```python
from build123d import *

# Parameters (mm, degrees)
BOSS_EXTRUDE1_DEPTH     = 8
BOSS_EXTRUDE2_DEPTH     = 2
SKETCH3_R               = 2.05
CUT_EXTRUDE3_DEPTH      = 10
CUT_EXTRUDE3_DEPTH_BACK = 10
FILLET2_R               = 4
SKETCH6_R               = 7.5
BOSS_EXTRUDE3_DEPTH     = 6
SKETCH2_R               = 5.5
CUT_EXTRUDE4_DEPTH      = 28.361360249
CUT_EXTRUDE4_DEPTH_BACK = 3
SKETCH8_R               = 0.8
CUT_EXTRUDE5_DEPTH      = 30.928860828
FILLET3_R               = 3


with BuildPart() as part:
    # Sketch1 → Boss-Extrude1 (new body)
    with BuildSketch(Plane(origin=(0, 0, 0), x_dir=(1, 0, 0), z_dir=(0, 1, 0))):
        Polygon((0, 0), (0, 2), (26.334414729, 2), (34.518104392, -15.549979118), (32.760161227, -16.503727422), (25.996962058, -2), (21.605779457, -2), (21.605779457, 0), align=None)
    extrude(amount=BOSS_EXTRUDE1_DEPTH)

    # Sketch5 → Boss-Extrude2 (add)
    with BuildSketch(Plane(origin=(22.396969556, 0, -10.443878423), x_dir=(-0.422618262, 0, -0.906307787), z_dir=(0.906307787, 0, -0.422618262))):
        with BuildLine():
            Line((-40.780850255, 18.736062391), (-36.467218683, 26.428860828))
            ThreePointArc((-36.467218683, 26.428860828), (-23.692308478, 4.771999965), (-36.205658542, -17.037035395))
            Line((-36.205658542, -17.037035395), (-40.049339329, -9.057253488))
            ThreePointArc((-40.049339329, -9.057253488), (-32.517126315, 5.047276383), (-40.780850255, 18.736062391))
        make_face()
    extrude(amount=-BOSS_EXTRUDE2_DEPTH)

    # Sketch3 → Cut-Extrude3 (cut, two sides)
    with BuildSketch(Plane(origin=(20.587699136, 0, -9.600201771), x_dir=(0.422618262, 0, 0.906307787), z_dir=(-0.906307787, 0, 0.422618262))) as cut_extrude3_sk:
        with Locations((28.701516689, 4)):
            Circle(SKETCH3_R)
        with Locations((34.117040182, 18.317355913)):
            Circle(SKETCH3_R)
        with Locations((48.070293023, 24.611901983)):
            Circle(SKETCH3_R)
        with Locations((62.387648936, 19.19637849)):
            Circle(SKETCH3_R)
        with Locations((68.682195005, 5.243125649)):
            Circle(SKETCH3_R)
        with Locations((63.266671512, -9.074230264)):
            Circle(SKETCH3_R)
        with Locations((49.313418672, -15.368776333)):
            Circle(SKETCH3_R)
        with Locations((34.996062759, -9.953252841)):
            Circle(SKETCH3_R)
    extrude(amount=CUT_EXTRUDE3_DEPTH, mode=Mode.SUBTRACT)
    extrude(cut_extrude3_sk.sketch, amount=-CUT_EXTRUDE3_DEPTH_BACK, mode=Mode.SUBTRACT)

    # Fillet2
    fillet2_edges = [part.edges().sort_by_distance(p)[0] for p in [
        (31.687047343, 0, 11.840592477),
        (31.60186373, 8, 11.657915631),
    ]]
    fillet(fillet2_edges, radius=FILLET2_R)

    # Sketch6 → Boss-Extrude3 (add)
    with BuildSketch(Plane(origin=(0, 0, -2), x_dir=(-1, 0, 0), z_dir=(0, 0, -1))):
        with Locations((0, 4)):
            Circle(SKETCH6_R)
    extrude(amount=-BOSS_EXTRUDE3_DEPTH)

    # Sketch2 → Cut-Extrude4 (cut, two sides)
    with BuildSketch(Plane.XY) as cut_extrude4_sk:
        with Locations((0, 4)):
            Circle(SKETCH2_R)
    extrude(amount=CUT_EXTRUDE4_DEPTH, mode=Mode.SUBTRACT)
    extrude(cut_extrude4_sk.sketch, amount=-CUT_EXTRUDE4_DEPTH_BACK, mode=Mode.SUBTRACT)

    # Sketch8 → Cut-Extrude5 (cut, through all)
    with BuildSketch(Plane(origin=(0, -3.5, 0), x_dir=(-1, 0, 0), z_dir=(0, -1, 0))):
        with Locations((0, -1.034043254)):
            Circle(SKETCH8_R)
    extrude(amount=-CUT_EXTRUDE5_DEPTH, mode=Mode.SUBTRACT)

    # Fillet3
    fillet3_edges = [part.edges().sort_by_distance(p)[0] for p in [
        (7.5, 4, 0),
    ]]
    fillet(fillet3_edges, radius=FILLET3_R)


solid = part.part
```
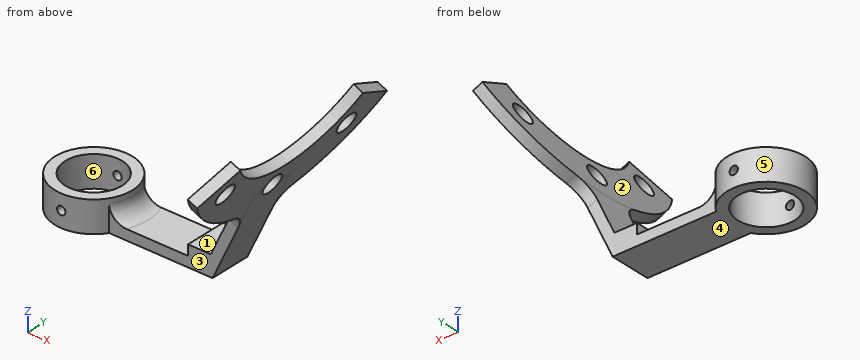
Part model, mm, in its own coordinate system. Face numbers are marked on the shaded views. A direction names the side the tool comes from. Coordinates: 2 decimals unless noted, no trailing zeros. Write each loop counter-clockwise with the first axis right and the second up, starting at its lowest first coordinate (ties: lowest second). Pieces come first, ordered by that corner, then holes.
Item 1: Slice it at A-A (x = 0). Write the cut outline in (y, z).
Item 2: Pin check, flat tips, straight feed: pin 1 (1.6 mm diameter, centred on y = 2, z = 1.5, fed in from -X); pin 2 (5 mm diameter, centred on x = 8, y = -5.5, fed in from -Z); pin 3 (5 mm diameter, centred on x = 24, y = 5.5, fed in from +Z); pin 4 (6 mm diameter, centred on y = 3, z = 19.5, fed in from -X). Stop position of each tip, or through.
Item 3: Slice it at B-B (y = 17). Write the cut outline in (x, z), and give its area (3 significant figures).
Item 4: Probe line 1 (X direction, y = 4, z = 2.25); line 2 (Z direction, x = 0, y = -3.1); line 3 (Y direction, x = 0, z = -0.5). List the from-to ranges inside material, lowest first.
Item 5: Mould opens along Y. For the marked faces 3, 4, 5 and 6 say: released by +Y, released by -Y, zero draft, split by the parting line, or undercut.
Item 6: Which spindle directions (+Z, -Z, +X, -X, +Y, -Y) get a long thin tool onto all of the face, cutting with end or side? Do the marked faces 1 and 2. Say none if no direction does.
Item 7: Slice it at C-C (y = 4). Count the separate pieces of the cut face and the enclosed holes in it, and give its area (3 significant figures).
Item 8: Slice it at D-D (z = 4.75). Write the cut outline in (x, y), and give its area (3 significant figures).
Results found:
1. outline: (-3.5, -2) - (-1.5, -2) - (-1.5, 0.23) - (-3.5, 0.23) - close; (-3.5, 1.83) - (-1.5, 1.83) - (-1.5, 4) - (-3.5, 4) - close; (9.5, -2) - (11.5, -2) - (11.5, 0.23) - (9.5, 0.23) - close; (9.5, 1.83) - (11.5, 1.83) - (11.5, 4) - (9.5, 4) - close
2. pin 1: stops at x = -7.4
2. pin 2: passes through
2. pin 3: stops at z = 3.08
2. pin 4: stops at x = 32.84
3. outline: (31.98, 14.85) - (33.8, 14) - (36.15, 19.05) - (34.34, 19.9) - close; (35.67, 22.75) - (37.48, 21.9) - (38.57, 24.24) - (36.76, 25.09) - close
3. area: 16.3 mm2
4. line 1: x = -7.5 to -5.5, 5.5 to 7.6, 26.11 to 28.32
4. line 2: z = -2 to 0.23, 1.83 to 4
4. line 3: y = -3.5 to -1.5, 9.5 to 11.5
5. face 3: released by -Y
5. face 4: zero draft
5. face 5: split by the parting line
5. face 6: undercut
6. face 1: +Z, +Y, -Y
6. face 2: +Z, -X, +Y, -Y
7. separate pieces: 3
7. enclosed holes: 0
7. area: 107 mm2
8. outline: (27.28, 0) - (29.48, 0) - (29.48, 8) - (27.28, 8) - close
8. area: 17.6 mm2
